```python
from build123d import *

# Parameters (mm, degrees)
F0_R     = 5
F0_R_2   = 3.5
F1_DEPTH = 10
F2_R     = 5
F3_DEPTH = 15
F3_TAPER = 14
F0_R_3   = 1
F4_DEPTH = 25.001


with BuildPart() as f1:
    # F0 (on Top) → F1 (new body)
    with BuildSketch(Plane.XY):
        Circle(F0_R)
        Circle(F0_R_2, mode=Mode.SUBTRACT)
    extrude(amount=F1_DEPTH)

    # F2 (on face) → F3 (join)
    with BuildSketch(Plane.XY.offset(10)):
        Circle(F2_R)
    extrude(amount=F3_DEPTH, taper=F3_TAPER)

    # F0 (on Top) → F4 (cut, through all)
    with BuildSketch(Plane.XY):
        Circle(F0_R_3)
    extrude(amount=F4_DEPTH, mode=Mode.SUBTRACT)


solid = f1.part
```
Work out the finished part from the listing and answer in its coordinate system (mm). A direction names the side the tool comes from. Coordinates: 2 decimals unless noted, no trailing zeros. Order: outer loops, then holes, each group sorted by start corner. A loop starts at its lowest first (then second) coordinate and runs counter-clockwise, first axis right, second up. Notation, with made-up numbers: M 53,59 L 106,59 A19 ccw 106,86 Z; hole C 4.5,52 d11. An arc over 180 degrees is marked long. Use CSV: the item, a comma, the result in double quotes.
1) Section D-D on z = 16.5 is taken. Write down the section's boundary in (x, y).
Worked out:
outline,"C 0,0 d6.76; hole C 0,0 d2"
2) Determine the mould class of faces 1 (the face through (3.233, -1.341, 4.93)), 2 (the face through (-1.08, -4.88, 4.93)), 3 (the face through (2.2, -3.3, 0)) for opening direction X: released by +X, released by -X, zero draft, split by the parting line, or undercut.
Worked out:
face 1,"undercut"
face 2,"split by the parting line"
face 3,"zero draft"
3) For faces 4 (the face through (1, -1, 10)), 5 (the face through (-0.67, -3.03, 17.6)), determine the directions among +Z, -Z, +X, -X, +Y, -Y from which every point of the face is accessible in a straight line to the end or side of a thin tool.
Worked out:
face 4,"-Z"
face 5,"+Z"
4) Section C-C on z = 5.75 is taken. Write down the section's boundary in (x, y), plus the area to 3 significant figures.
Worked out:
outline,"C 0,0 d10; hole C 0,0 d7"
area,"40.1 mm^2"
5) Section A-A on y = 0 is taken. Write down the section's boundary in (x, z).
Worked out:
outline,"M -5,0 L -3.5,0 L -3.5,10 L -1,10 L -1,25 L -1.26,25 L -5,10 Z; M 1,10 L 3.5,10 L 3.5,0 L 5,0 L 5,10 L 1.26,25 L 1,25 Z"
6) Consider line 1 (Y direction, x = 0, z = 5.75); line 2 (X direction, y = 2.25, z = 7.25); line 3 (Y direction, x = 0, z = 16). Determine where each line is inside the solid, lowest interval first. Write a range as [from, to].
Worked out:
line 1,"y = [-5, -3.5], [3.5, 5]"
line 2,"x = [-4.47, -2.68], [2.68, 4.47]"
line 3,"y = [-3.5, -1], [1, 3.5]"
7) Flat-ended cylindrical pins translate along their axes: pin 1 Ø4 at (x, z) = (-1, 12.5) entering from +Y; pin 2 Ø6 at (x, z) = (-0.5, 17.5) entering from +Y; pin 3 Ø2 at (x, y) = (0.5, -1.5) entering from -Z. Find the tip coordinate at first contact, or state that the pin passes through.
Worked out:
pin 1,"stops at y = 4.84"
pin 2,"stops at y = 3.87"
pin 3,"stops at z = 10"
